Source: CAD feature listing. Evaluate the final solid. Frame: model axes, mm. A direction names the side the tool comes from. Coordinates: 2 decimals unless noted, no trailing zeros. Order: outer loops, then holes, each group sorted by start corner. A loop starts at its lowest first (then second) coordinate and runs counter-clockwise, first axis right, second up.
Autodesk Inventor part; units mm, degrees
ref_plane "Work Plane1" through (-41.91, 0, -101.6) normal (-1, 0, 0) x (0, 0, 1)
ref_plane "Work Plane2" through (-48.26, 0, -101.6) normal (-1, 0, 0) x (0, 0, 1)
ref_plane "YZ Plane" through (0, 0, 0) normal (1, 0, 0) x (0, 1, 0)
sketch "Sketch1" plane through (0, 0, 0) normal (0, 1, 0) x (-1, 0, 0)
  line L0 (0, 0) -> (41.91, 0)
  line L1 (41.91, 0) -> (41.91, -127)
  line L2 (41.91, -127) -> (0, -127)
  line L3 (0, -127) -> (0, 0)
  dimension "d0" = 127
  dimension "d1" = 41.91
extrude "Extrusion1" add sketch "Sketch1" along normal blind 6.35
sketch "Sketch2" plane through (0, 6.35, 0) normal (0, 1, 0) x (1, 0, 0)
  line L0 (-25.4, 26.035) -> (-21.59, 26.035)
  line L1 (-21.59, 26.035) -> (-21.59, 30.48)
  line L2 (-21.59, 30.48) -> (-25.4, 30.48)
  line L3 (-25.4, 30.48) -> (-25.4, 26.035)
  line L4 (-25.4, 96.52) -> (-21.59, 96.52)
  line L5 (-21.59, 96.52) -> (-21.59, 100.965)
  line L6 (-21.59, 100.965) -> (-25.4, 100.965)
  line L7 (-25.4, 100.965) -> (-25.4, 96.52)
  line L8 (0, 0) -> (0, 127)
  line L9 (-41.91, 0) -> (0, 0)
  line L10 (0, 127) -> (-41.91, 127)
  line L11 (-17.018, 26.035) -> (-13.208, 26.035)
  line L12 (-13.208, 26.035) -> (-13.208, 30.48)
  line L13 (-13.208, 30.48) -> (-17.018, 30.48)
  line L14 (-17.018, 30.48) -> (-17.018, 26.035)
  line L15 (-17.018, 96.52) -> (-13.208, 96.52)
  line L16 (-13.208, 96.52) -> (-13.208, 100.965)
  line L17 (-13.208, 100.965) -> (-17.018, 100.965)
  line L18 (-17.018, 100.965) -> (-17.018, 96.52)
  line L19 (-41.91, 127) -> (-41.91, 0)
  dimension "d5" = 4.445
  dimension "d6" = 3.81
  dimension "d7" = 4.445
  dimension "d8" = 26.035
  dimension "d9" = 26.035
  dimension "d12" = 4.445
  dimension "d13" = 4.445
  dimension "d14" = 3.81
  dimension "d15" = 26.035
  dimension "d16" = 26.035
  dimension "d18" = 8.382
  dimension "d36" = 16.51
extrude "Extrusion3" cut sketch "Sketch2" against normal blind 6.35 contours L3 L2 L1 L0 | L7 L6 L5 L4 | L14 L13 L12 L11 | L18 L17 L16 L15
sketch "Sketch4" plane through (0, 6.35, 0) normal (0, 1, 0) x (1, 0, 0)
  line L0 (-41.91, 127) -> (-41.91, 0)
  line L1 (-41.91, 114.3) -> (-29.21, 114.3)
  line L2 (-29.21, 114.3) -> (-29.21, 12.7)
  line L3 (-29.21, 12.7) -> (-41.91, 12.7)
  line L4 (-41.91, 12.7) -> (-41.91, 114.3)
  line L5 (-41.91, 0) -> (0, 0)
  line L6 (0, 127) -> (-41.91, 127)
  dimension "d61" = 12.7
  dimension "d62" = 12.7
  dimension "d63" = 12.7
sketch "Sketch6" plane through (0, 6.35, 0) normal (0, 1, 0) x (1, 0, 0)
  line L0 (0, 127) -> (-41.91, 127)
  line L1 (-40.3225, 127) -> (-37.1475, 127)
  line L2 (-37.1475, 127) -> (-37.1475, 120.65)
  line L3 (-37.1475, 120.65) -> (-40.3225, 120.65)
  line L4 (-40.3225, 120.65) -> (-40.3225, 127)
  line L5 (-41.91, 0) -> (0, 0)
  line L6 (-40.3225, 0) -> (-37.1475, 0)
  line L7 (-37.1475, 0) -> (-37.1475, 6.35)
  line L8 (-37.1475, 6.35) -> (-40.3225, 6.35)
  line L9 (-40.3225, 6.35) -> (-40.3225, 0)
  line L10 (-41.91, 127) -> (-41.91, 0)
  point P0 (-41.91, 107.95)
  dimension "d37" = 1.5875
  dimension "d38" = 6.35
  dimension "d39" = 3.175
  dimension "d40" = 6.35
extrude "Extrusion6" cut sketch "Sketch6" against normal blind 25.4
ref_plane "Work Plane1" through (-41.91, 0, -101.6) normal (-1, 0, 0) x (0, 0, 1)
sketch "Sketch7" plane through (-41.91, 0, -101.6) normal (-1, 0, 0) x (0, 0, 1)
  line L0 (88.9, 6.35) -> (88.9, 0)
  line L1 (101.6, 0) -> (101.6, 6.35)
  line L2 (88.9, 6.35) -> (101.6, 6.35)
  line L3 (101.6, 6.35) -> (101.6, 0)
  line L4 (101.6, 0) -> (88.9, 0)
  line L5 (88.9, 0) -> (88.9, 6.35)
  line L6 (101.6, 0) -> (-25.4, 0)
  line L7 (-25.4, 6.35) -> (-12.7, 6.35)
  line L8 (-12.7, 6.35) -> (-12.7, 0)
  line L9 (-12.7, 0) -> (-25.4, 0)
  line L10 (-25.4, 0) -> (-25.4, 6.35)
  point P0 (-6.35, 0)
  point P1 (-19.05, 6.35)
  dimension "d66" = 12.7
extrude "Extrusion10" add sketch "Sketch7" along normal blind 6.35
ref_plane "Work Plane2" through (-48.26, 0, -101.6) normal (-1, 0, 0) x (0, 0, 1)
extrude "Extrusion9" cut sketch "Sketch4" against normal blind 6.35
sketch "Sketch10" plane through (-48.26, 0, -101.6) normal (-1, 0, 0) x (0, 0, 1)
  line L0 (95.25, 0) -> (92.075, 0)
  line L1 (92.075, 0) -> (92.075, 6.35)
  line L2 (92.075, 6.35) -> (95.25, 6.35)
  line L3 (95.25, 6.35) -> (95.25, 0)
  line L4 (-19.05, 0) -> (-15.875, 0)
  line L5 (-15.875, 0) -> (-15.875, 6.35)
  line L6 (-15.875, 6.35) -> (-19.05, 6.35)
  line L7 (-19.05, 6.35) -> (-19.05, 0)
  line L8 (-25.4, 6.35) -> (-25.4, 0)
  line L9 (101.6, 0) -> (101.6, 6.35)
  point P0 (-12.7, 0)
  dimension "d70" = 3.175
  dimension "d72" = 3.175
  dimension "d73" = 6.35
  dimension "d74" = 6.35
  dimension "d75" = 6.35
  dimension "d76" = 6.35
extrude "Extrusion12" cut sketch "Sketch10" against normal blind 6.35
sketch "Sketch11" plane through (0, 6.35, 0) normal (0, 1, 0) x (1, 0, 0)
  line L0 (-11.43, 60.96) -> (-5.08, 60.96)
  line L1 (-5.08, 60.96) -> (-5.08, 54.61)
  line L2 (-5.08, 54.61) -> (-11.43, 54.61)
  line L3 (-11.43, 54.61) -> (-11.43, 60.96)
  line L4 (-37.1475, 0) -> (0, 0)
  line L5 (0, 0) -> (0, 127)
  line L6 (-29.21, 114.3) -> (-29.21, 12.7)
  dimension "d82" = 54.61
  dimension "d83" = 6.35
  dimension "d84" = 6.35
  dimension "d86" = 17.78
extrude "Extrusion13" cut sketch "Sketch11" against normal blind 6.35
sketch "Sketch12" plane through (0, 6.35, 0) normal (0, 1, 0) x (1, 0, 0)
  line L0 (-22.86, 50.673) -> (-16.51, 50.673)
  line L1 (-16.51, 50.673) -> (-16.51, 57.023)
  line L2 (-16.51, 57.023) -> (-22.86, 57.023)
  line L3 (-22.86, 57.023) -> (-22.86, 50.673)
  line L4 (-22.86, 69.977) -> (-16.51, 69.977)
  line L5 (-16.51, 69.977) -> (-16.51, 76.327)
  line L6 (-16.51, 76.327) -> (-22.86, 76.327)
  line L7 (-22.86, 76.327) -> (-22.86, 69.977)
  line L8 (-29.21, 114.3) -> (-29.21, 12.7)
  line L9 (-37.1475, 0) -> (0, 0)
  line L10 (0, 127) -> (-37.1475, 127)
  dimension "d90" = 6.35
  dimension "d91" = 6.35
  dimension "d92" = 6.35
  dimension "d93" = 50.673
  dimension "d94" = 6.35
  dimension "d95" = 50.673
extrude "Extrusion14" cut sketch "Sketch12" against normal blind 6.35
sketch "Sketch13" plane through (-29.21, 6.35, -114.3) normal (-1, 0, 0) x (0, 0, 1)
  line L0 (101.6, -6.35) -> (63.5, -6.35)
  line L1 (63.5, -6.35) -> (63.5, 0)
  line L2 (63.5, 0) -> (101.6, 0)
  line L3 (101.6, 0) -> (101.6, -6.35)
  line L4 (101.6, -6.35) -> (0, -6.35)
  line L5 (0, 0) -> (101.6, 0)
  line L6 (0, -6.35) -> (38.1, -6.35)
  line L7 (38.1, -6.35) -> (38.1, 0)
  line L8 (38.1, 0) -> (0, 0)
  line L9 (0, 0) -> (0, -6.35)
  point P0 (114.3, -6.35)
  dimension "d98" = 38.1
  dimension "d99" = 38.1
extrude "Extrusion15" add sketch "Sketch13" along normal blind 1.27 contours L0 L1 L2 L3 | L4 L9 L5 L7
properties part number "MonsterHolderBase"
Q1. Set-up query: faces 1 (the flat face through (-20, 3, -50.673)), 2 (the flat face through (-37.148, 3, -124)), 3 (the flat face through (-29.21, 3, -64)). Return all of +Z, -Z, +X, -X, +Y, -Y with unobstructed straight access to the full face (end or side cutting, diameter ignored); none if empty.
Solutions:
face 1: +Y, -Y
face 2: -Z, +Y, -Y
face 3: -X, +Y, -Y
Q2. Section query C-C on z = -109. Output: boundary loops of the cut face in (x, y).
Solutions:
outline: (-30.48, 0) - (0, 0) - (0, 6.35) - (-30.48, 6.35) - close
Q3. Section query B-B on y = 3. Give the number of separate pieces and of enclosed holes in the cut face, plus the area to 3 significant figures.
Solutions:
separate pieces: 1
enclosed holes: 7
area: 4,020 mm2
Q4. Material intervals for line 1 along Z through (x, y) = (-15, 3) (3 decimals); line 2 along Z through (x, y) = (-42.5, 1.25) (3 decimals); line 3 along X through (y, z) = (2, -55), sorted ascending.
Solutions:
line 1: z = -127 to -100.965, -96.52 to -30.48, -26.035 to 0
line 2: z = -127 to -120.65, -117.475 to -114.3, -12.7 to -9.525, -6.35 to 0
line 3: x = -29.21 to -22.86, -16.51 to -11.43, -5.08 to 0
Q5. Pin query (flat end, axial travel): P1, Ø2, axis at y = 3, z = -80.5, coming from the -X side; P2, Ø1.9, axis at y = 4, z = -69.5, coming from the -X side. Return the tip coordinate at first contact, or that it passes through.
Solutions:
P1: stops at x = -30.48
P2: stops at x = -29.21
Q6. Pull-direction query (X, two-part tool) for faces 4 (the flat face through (-18, 0, -63)), 5 (the flat face through (-20, 3, -57.023)), 6 (the flat face through (-48.26, 3, -3)); classes: pulls with the +X half, pulls with the -X half, needs draft (parallel to the pull), parting line crosses it, or undercut.
Solutions:
face 4: needs draft
face 5: undercut
face 6: pulls with the -X half
Q7. Section query A-A on z = -53. Output: boundary loops of the cut face in (x, y).
Solutions:
outline: (-29.21, 0) - (-22.86, 0) - (-22.86, 6.35) - (-29.21, 6.35) - close; (-16.51, 0) - (0, 0) - (0, 6.35) - (-16.51, 6.35) - close
